```python
from build123d import *

# Parameters (mm, degrees)
F0_W        = 1400
F0_H        = 790
F1_DEPTH    = 30
F2_W        = 1398
F2_H        = 510
F3_DEPTH    = 28
F4_W        = 500
F4_H        = 400
F5_DEPTH    = 300
F6_T        = 2
F6_T3_DEPTH = 404
F6_T5_DEPTH = 504
F6_T7_DEPTH = 32
F7_R        = 50
F8_R        = 25
F9_DEPTH    = 2
F10_R       = 15
F10_R_2     = 20
F11_DEPTH   = 30
F12_W       = 510
F12_H       = 2
F13_DEPTH   = 5
F14_W       = 510
F14_H       = 2
F15_ANGLE   = 90
F16_W       = 2
F16_H       = 510
F17_DEPTH   = 10
F18_W       = 30
F18_H       = 30
F19_DEPTH   = 850
F20_W       = 30
F20_H       = 30
F21_DEPTH   = 1200
F22_W       = 30
F22_H       = 30
F23_DEPTH   = 545
F25_DEPTH   = 2
F27_DEPTH   = 400
F28_R       = 75


# Not quite as in the source:
# - a shell that OpenCascade refuses in one call is made with other operations: the cavity is built on its own and cut out


with BuildPart() as f1:
    # F0 (on Top) → F1 (new body)
    with BuildSketch(Plane.XY):
        with Locations((700, 395)):
            Rectangle(F0_W, F0_H)
    extrude(amount=F1_DEPTH)

    # F2 (on face) → F3 (cut)
    with BuildSketch(Plane.XY.offset(30)):
        with Locations((701, 285)):
            Rectangle(F2_W, F2_H)
    extrude(amount=-F3_DEPTH, mode=Mode.SUBTRACT)

    # F4 (on face) → F5 (join)
    with BuildSketch(Plane(origin=(0, 0, 0), x_dir=(1, 0, 0), z_dir=(0, 0, -1))):
        with Locations((370, -285)):
            Rectangle(F4_W, F4_H)
    extrude(amount=F5_DEPTH)

    # F6: shell of thickness 2, made by hand


with BuildPart() as f6_core1:
    # F6_t2: copy of F1
    add(f1.part)

    # the walls: a layer under each face that stays
    f6_faces = [f6_core1.faces().sort_by_distance(p)[0] for p in [
        (0, 395, 15),
        (700, 790, 15),
        (700, 0, 15),
        (700, 395, 0),
        (233.3333333333, 658.3333333333, 30),
        (1400, 658.3333333333, 25),
        (620, 285, -150),
        (370, 485, -150),
        (120, 285, -150),
        (370, 85, -150),
        (701, 540, 16),
        (2, 285, 16),
        (701, 30, 16),
        (370, 285, -300),
    ]]
    thicken(f6_faces, amount=-F6_T, mode=Mode.SUBTRACT)

    # F6_s4 → F6_t3 (cut)
    with BuildSketch(Plane.XZ.offset(-487)):
        Polygon((620.02, -0.02), (620, 2), (618, 2), (618, 0), align=None)
        Polygon((119.98, -0.02), (120, 2), (122, 2), (122, 0), align=None)
    extrude(amount=F6_T3_DEPTH, mode=Mode.SUBTRACT)

    # F6_s6 → F6_t5 (cut)
    with BuildSketch(Plane.YZ.offset(118)):
        Polygon((485.02, -0.02), (485, 2), (483, 2), (483, 0), align=None)
        Polygon((84.98, -0.02), (85, 2), (87, 2), (87, 0), align=None)
    extrude(amount=F6_T5_DEPTH, mode=Mode.SUBTRACT)

    # F6_s8 → F6_t7 (cut)
    with BuildSketch(Plane.XY):
        Polygon((2.02, 539.98), (2, 542), (0, 542), (0, 540), align=None)
        Polygon((2.02, 30.02), (0, 30), (0, 28), (2, 28), align=None)
    extrude(amount=F6_T7_DEPTH, mode=Mode.SUBTRACT)


with BuildPart() as f1_1:
    add(f1.part)

    # what is left inside the walls is the cavity
    f6_cavity = [f6_core1.part.solids().sort_by_distance(p)[0] for p in [
        (700, 10.666667, 2.02),
        (700, 624, 27.98),
        (370, 351, -297.98),
    ]]
    add(f6_cavity, mode=Mode.SUBTRACT)

    # F7
    f7_edges = [f1_1.edges().sort_by_distance(p)[0] for p in [
        (122, 483, -148),
        (618, 483, -148),
        (122, 87, -148),
        (618, 87, -148),
        (618, 285, -298),
        (370, 483, -298),
        (122, 285, -298),
        (370, 87, -298),
        (120, 85, -150),
        (370, 85, -300),
        (620, 85, -150),
        (620, 285, -300),
        (620, 485, -150),
        (370, 485, -300),
        (120, 485, -150),
        (120, 285, -300),
    ]]
    fillet(f7_edges, radius=F7_R)

    # F8 (on face) → F9 (cut, through all)
    with BuildSketch(Plane.XY.offset(-298)):
        with Locations((488, 353)):
            Circle(F8_R)
    extrude(amount=-F9_DEPTH, mode=Mode.SUBTRACT)

    # F10 (on face) → F11 (cut, through all)
    with BuildSketch(Plane.XY.offset(30)):
        with Locations((550, 665)):
            Circle(F10_R)
        with Locations((370, 665)):
            Circle(F10_R)
        with Locations((190, 665)):
            Circle(F10_R_2)
    extrude(amount=-F11_DEPTH, mode=Mode.SUBTRACT)

    # F12 (on face) → F13 (join)
    with BuildSketch(Plane.YZ.offset(1400)):
        with Locations((285, 1)):
            Rectangle(F12_W, F12_H)
    extrude(amount=F13_DEPTH)

    # F14 (on face) → F15 (revolve)
    with BuildSketch(Plane.YZ.offset(1405)):
        with Locations((285, 1)):
            Rectangle(F14_W, F14_H)
    revolve(axis=Axis((1405, 285, 0), (0, 1, 0)), revolution_arc=F15_ANGLE)

    # F16 (on face) → F17 (join)
    with BuildSketch(Plane(origin=(0, 0, 0), x_dir=(1, 0, 0), z_dir=(0, 0, -1))):
        with Locations((1406, -285)):
            Rectangle(F16_W, F16_H)
    extrude(amount=F17_DEPTH)

    # F18 (on face) → F19 (join)
    with BuildSketch(Plane(origin=(0, 0, 0), x_dir=(1, 0, 0), z_dir=(0, 0, -1))):
        with Locations((85, -45)):
            Rectangle(F18_W, F18_H)
        with Locations((1315, -45)):
            Rectangle(F18_W, F18_H)
        with Locations((1315, -620)):
            Rectangle(F18_W, F18_H)
        with Locations((85, -620)):
            Rectangle(F18_W, F18_H)
    extrude(amount=F19_DEPTH)

    # F20 (on face) → F21 (join, through all)
    with BuildSketch(Plane.YZ.offset(100)):
        with Locations((45, -715)):
            Rectangle(F20_W, F20_H)
        with Locations((620, -715)):
            Rectangle(F20_W, F20_H)
    extrude(amount=F21_DEPTH)

    # F22 (on face) → F23 (join, through all)
    with BuildSketch(Plane(origin=(0, 60, 0), x_dir=(-1, 0, 0), z_dir=(0, 1, 0))):
        with Locations((-1315, -715)):
            Rectangle(F22_W, F22_H)
        with Locations((-85, -715)):
            Rectangle(F22_W, F22_H)
    extrude(amount=F23_DEPTH)

    # F24 (on face) → F25 (join)
    with BuildSketch(Plane.XY.offset(-700)):
        Polygon((100, 60), (100, 30), (1300, 30), (1300, 60), (1330, 60), (1330, 605), (1300, 605), (1300, 635), (100, 635), (100, 605), (70, 605), (70, 60), align=None)
    extrude(amount=F25_DEPTH)

    # F26 (on face) → F27 (join)
    with BuildSketch(Plane.XY.offset(30)):
        Polygon((1400, 790), (0, 790), (0, 540), (2, 540), (2, 788), (1398, 788), (1398, 540), (1400, 540), align=None)
    extrude(amount=F27_DEPTH)

    # F28
    f28_edges = [f1_1.edges().sort_by_distance(p)[0] for p in [
        (1, 540, 430),
        (1399, 540, 430),
    ]]
    fillet(f28_edges, radius=F28_R)


solid = f1_1.part
```
Check sheet for the modelled part. Datum: model origin and axes. Units: mm. A direction names the side the tool comes from. Give positions to 0.01 mm unless a question says otherwise; leave off trailing zeros. Write each loop counter-clockwise with the first axis right and the second up, starting at its lowest first coordinate (ties: lowest second). Pieces come first, ordered by that corner, then holes. Notation, with made-up numbers: (-25, -0.5) - (7, -0.5) arc R28 ccw to (7, 24.5) - close; hole circle Ø11 at (-23.5, 19.25). An arc over 180 degrees is marked (long way). Answer as a JSON object with one key per item and string values. Group by question number.
1) Sectioned sample at B-B (y = 507.5). Record the cut outline in (x, z).
2) Access from +Z, -Z, +X, -X, +Y, -Y to the whole of each face (thin tool, end or side, straight path). Record for faces 1 (the face through (372.772, 101.258, -282.964)), 2 (the face through (690, 666, 30)), 3 (the face through (690, 667, 2)).
3) Sectioned sample at D-D (y = 353). Give the number of separate pieces and of enclosed holes in the cut face, then the cut area to 3 significant figures.
4) Depth check by flat-ended pin: P1, Ø24, axis at x = 1315.5, z = -461, coming from the +Y side; P2, Ø8, axis at x = 941, y = 141.5, coming from the -Z side; P3, Ø5, axis at x = 607, y = 469, coming from the +Z side. Enter the tip coordinate at first touch or a pass-through.
5) Thickness scan on probe 1 along Z at (x, y) = (1006.5, 576); probe 2 along X at (y, z) = (39, -438); probe 3 along Z at (x, y) = (1328, 655.5). Record the ranges inside material, lowest first. Write a range as from..to.
6) Release check for a two-part mould opening along X. For faces 4 (the face through (134.258, 469.964, -126.75)), 5 (the face through (1399.01, 561.39, 407.45)), 6 (the face through (187.4, 684.83, 1.01)) record: pulls with the +X half, pulls with the -X half, needs draft (parallel to the pull), parting line crosses it, or undercut.
7) Sectioned sample at C-C (z = -474.5). Record the cut outline in (x, y), then the cut area to 3 significant figures.
8) Sectioned sample at A-A (x = 1101). Record the cut outline in (y, z), then the cut area to 3 significant figures.
Geometry results:
{
 "1": {"outline": "(0, 0) - (1405, 0) - (1405, -10) - (1407, -10) - (1407, 0) arc R2 ccw to (1405, 2) - (2, 2) - (2, 30) - (0, 30) - close; (70, -730) - (100, -730) - (100, -700) - (1300, -700) - (1300, -730) - (1330, -730) - (1330, -698) - (70, -698) - close"},
 "2": {"face 1": "+Z", "face 2": "+Z, -Y", "face 3": "none"},
 "3": {"separate pieces": "3", "enclosed holes": "0", "area": "8,310 mm^2"},
 "4": {"P1": "stops at y = 635", "P2": "stops at z = -700", "P3": "stops at z = 2"},
 "5": {"probe 1": "z = -700..-698, 0..2, 28..30", "probe 2": "x = 70..100, 1300..1330", "probe 3": "z = 0..2, 28..30"},
 "6": {"face 4": "pulls with the -X half", "face 5": "needs draft", "face 6": "undercut"},
 "7": {"outline": "(70, 30) - (100, 30) - (100, 60) - (70, 60) - close; (70, 605) - (100, 605) - (100, 635) - (70, 635) - close; (1300, 30) - (1330, 30) - (1330, 60) - (1300, 60) - close; (1300, 605) - (1330, 605) - (1330, 635) - (1300, 635) - close", "area": "3,600 mm^2"},
 "8": {"outline": "(0, 0) - (790, 0) - (790, 430) - (788, 430) - (788, 30) - (540, 30) - (540, 2) - (30, 2) - (30, 30) - (0, 30) - close; (30, -730) - (60, -730) - (60, -700) - (605, -700) - (605, -730) - (635, -730) - (635, -698) - (30, -698) - close; hole (2, 2) - (28, 2) - (28, 28) - (2, 28) - close; hole (542, 2) - (788, 2) - (788, 28) - (542, 28) - close", "area": "6,160 mm^2"}
}
